Study the drawing (mm; zero at the part's minimum x, y, z) and answer. A direction names the side the tool comes from. Round coordinates to 2 decimals unless told otherwise and drop trailing zeros. Loops run counter-clockwise (first coordinate to the right, second up) from the corner with the lowest first, then second, coordinate; pieces in that order, holes last. Notation, with made-up numbers: M 32,53.5 L 60,53.5 A25 ccw 60,84.5 Z; hole C -36.5,53.5 d2. An arc over 180 degrees is marked long. Put each result on its own line as item: value. Start each with the question number.
(1) Section B-B, the plane z = 248.5 is taken. Determine the outline of the cut face in (x, y).
(2) Flat-ended cylindrical pins translate along their axes: P1, Ø6, axis at x = 338.5, z = 416.5, coming from the -Y side; P2, Ø4, axis at x = 513, y = 536, coming from the -Z side; P3, Ø2, axis at x = 278, z = 165, coming from the +Y side. Find the tip coordinate at first contact, or state that the pin passes through.
(3) Section A-A, the plane y = 502 is taken. Determine the outline of the cut face in (x, z).
(4) Section D-D, the plane z = 96 is taken. Determine the outline of the cut face in (x, y), then the cut area to 3 significant figures.
(5) Straight lines are drawn through the part: line 1 (Z direction, x = 181.5, y = 322); line 2 (X direction, y = 362.5, z = 330); line 3 (Y direction, x = 303, z = 343). For each, find the intervals that lie inside material, in ascending order.
(6) Determine the mould class of the marked faces 3, 4 and 5 for opening direction Z: released by +Z, released by -Z, zero draft, split by the parting line, or undercut.
(7) Section C-C, the plane x = 497.5 is taken. Determine the outline of the cut face in (y, z), then the cut area to 3 significant figures.
(8) Which of the six approach directions +Z, -Z, +X, -X, +Y, -Y give full straight-line access (tool end or side, diameter ignored) to the marked faces 1 and 2?
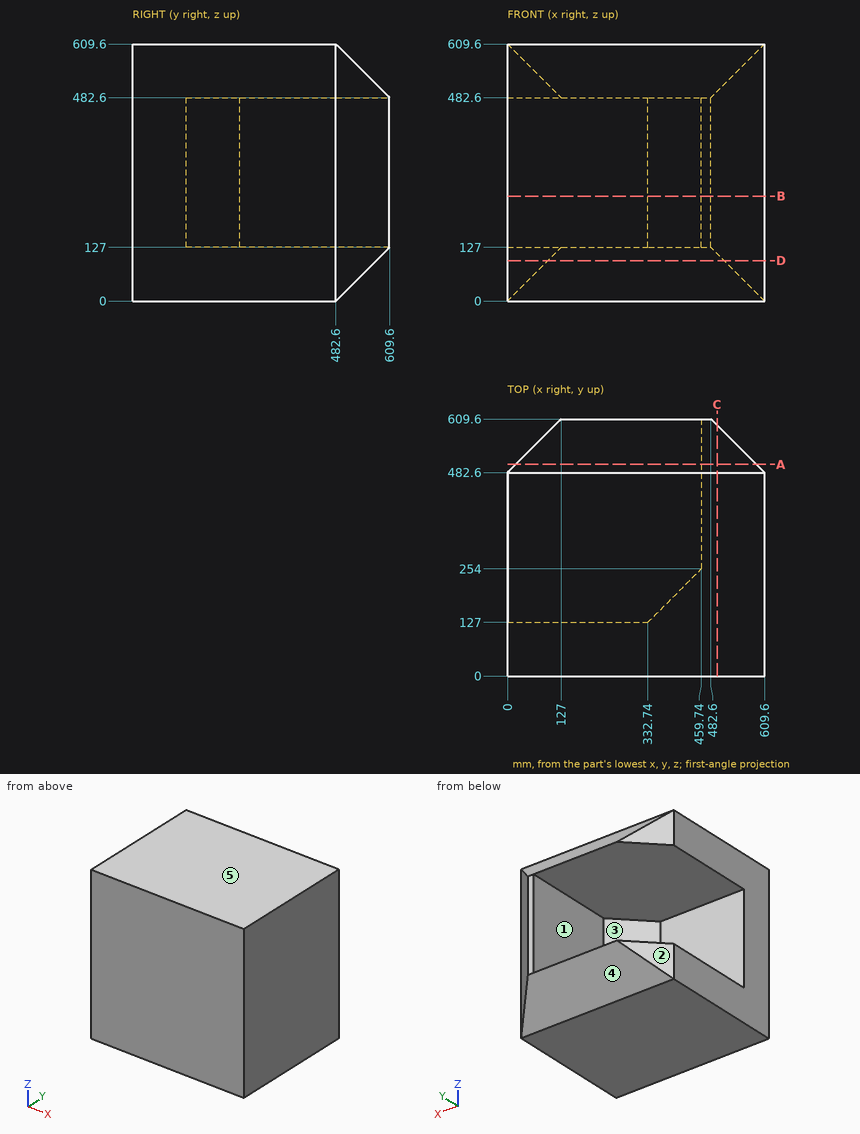
Recorded:
1. outline: M 0,0 L 609.6,0 L 609.6,482.6 L 482.6,609.6 L 459.74,609.6 L 459.74,254 L 332.74,127 L 0,127 Z
2. P1: stops at y = 0
2. P2: stops at z = 51.4
2. P3: stops at y = 127
3. outline: M 19.4,19.4 L 590.2,19.4 L 590.2,590.2 L 19.4,590.2 L 19.4,482.6 L 459.74,482.6 L 459.74,127 L 19.4,127 Z
4. outline: M 0,0 L 609.6,0 L 609.6,482.6 L 513.6,578.6 L 96,578.6 L 0,482.6 Z
4. area: 343,000 mm²
5. line 1: z = 0 to 127, 482.6 to 609.6
5. line 2: x = 459.74 to 609.6
5. line 3: y = 0 to 127
6. face 3: undercut
6. face 4: released by -Z
6. face 5: released by +Z
7. outline: M 0,0 L 482.6,0 L 594.7,112.1 L 594.7,497.5 L 482.6,609.6 L 0,609.6 Z
7. area: 350,000 mm²
8. face 1: -X, +Y
8. face 2: +Z, -Z, -X, +Y
